Can you work these out from the model? Positions are in its coordinate system, mm. A direction names the side the tool comes from. Round coordinates to 2 decimals unless told otherwise and drop trailing zeros. Write each loop counter-clockwise with the first axis right and the second up, starting at its lowest first coordinate (ties: lowest second). Pieces come first, ordered by that corner, then holes.
Q1. For faces 1 (the flat face through (0, 37.5, 13)), 2 (the flat face through (14.5, 1, 5)), 3 (the flat face through (-14, -39.5, 7)), which set-ups out of +Z, -Z, +X, -X, +Y, -Y let a thin tool reach every point of the face, with its end or its side?
Q2. I'm going to push flat-ended pins straight in: pin 1 Ø1.6 at (x, y) = (-13.5, -1) entering from +Z; pin 2 Ø10 at (x, y) = (4.5, 19) entering from +Z; pin 3 Ø1.2 at (x, z) = (-8.47, 12.5) entering from -Y; pin 4 Ø1 at (x, z) = (-13, 6) entering from -Y. Where does each tip first touch, or does it pass through?
Q3. Please list where these lines run through material, in increasing order: line 1 along Y through (x, z) = (0, -0.55); line 2 along X through (y, z) = (7, 5.5); line 3 along Z through (x, y) = (1.75, 24.5).
Q4. If we section it at A-A (y = 34.5): Please give me the cut outline in (x, z).
Q5. We'd pull the mould along X, two halves only. Please class faces 4 (the cylindrical face through (0, -48, -1)), 5 (the flat face through (14, -39.5, 7)), 6 (the flat face through (-14.5, 1, 5)): +X half, -X half, draft (parallel to the pull), parting line (faces both ways), or undercut.
Q6. If we section it at B-B (x = 0): Please give me the cut outline in (y, z), plus the area to 3 significant figures.
Q7. If we section it at C-C (z = 10): Please give me the cut outline in (x, y), plus the area to 3 significant figures.
Q8. If we section it at D-D (x = 8.5): Please give me the cut outline in (y, z).
from build123d import *

# Parameters (mm, degrees)
ESQUISSE1_R             = 1
BOSS_EXTRU_2_DEPTH      = 2
ESQUISSE4_W             = 12.5
ESQUISSE4_H             = 79
BOSS_EXTRU_3_DEPTH      = 2
ESQUISSE6_W             = 12.5
ESQUISSE6_H             = 79
BOSS_EXTRU_4_DEPTH      = 2
BOSS_EXTRU_7_DEPTH      = 2
ESQUISSE14_R            = 1
ENL_V_MAT_EXTRU_4_DEPTH = 98.864702523
CHANFREIN3_SIZE         = 0.5
CONG_1_R                = 1


with BuildPart() as part:
    # Esquisse1 → Boss.-Extru.2 (new body)
    with BuildSketch(Plane.XY):
        with BuildLine():
            Line((14.5, -39.5), (14.5, 39.5))
            Line((14.5, 39.5), (-14.5, 39.5))
            Line((-14.5, 39.5), (-14.5, -39.5))
            ThreePointArc((-14.5, -39.5), (0, -54), (14.5, -39.5))
        make_face()
        with Locations((0, 34.5)):
            Circle(ESQUISSE1_R, mode=Mode.SUBTRACT)
        with Locations((0, -49)):
            Circle(ESQUISSE1_R, mode=Mode.SUBTRACT)
    extrude(amount=-BOSS_EXTRU_2_DEPTH)

    # Esquisse4 → Boss.-Extru.3 (add)
    with BuildSketch(Plane.ZY.offset(14.5)):
        with Locations((6.25, 0)):
            Rectangle(ESQUISSE4_W, ESQUISSE4_H)
    extrude(amount=-BOSS_EXTRU_3_DEPTH)

    # Esquisse6 → Boss.-Extru.4 (add)
    with BuildSketch(Plane(origin=(14.5, 0, 0), x_dir=(0, 0, -1), z_dir=(1, 0, 0))):
        with Locations((-6.25, 0)):
            Rectangle(ESQUISSE6_W, ESQUISSE6_H)
    extrude(amount=-BOSS_EXTRU_4_DEPTH)

    # Esquisse11 → Boss.-Extru.7 (add)
    with BuildSketch(Plane(origin=(0, 39.5, 0), x_dir=(1, 0, 0), z_dir=(0, 1, 0))):
        with BuildLine():
            Line((-12.5, 0), (12.5, 0))
            Line((12.5, 0), (12.5, -12.5))
            ThreePointArc((12.5, -12.5), (0, -25), (-12.5, -12.5))
            Line((-12.5, -12.5), (-12.5, 0))
        make_face()
    extrude(amount=-BOSS_EXTRU_7_DEPTH)

    # Esquisse14 → Enlèv. mat.-Extru.4 (cut, through all)
    with BuildSketch(Plane(origin=(0, 39.5, 0), x_dir=(1, 0, 0), z_dir=(0, 1, 0))):
        with Locations(Location((-8.474453363, -12.5, 0), (0, 0, 270))):
            Circle(ESQUISSE14_R)
        with Locations(Location((8.5, -12.5, 0), (0, 0, 270))):
            Circle(ESQUISSE14_R)
    extrude(amount=-ENL_V_MAT_EXTRU_4_DEPTH, mode=Mode.SUBTRACT)

    # Chanfrein3
    chanfrein3_edges = [part.edges().sort_by_distance(p)[0] for p in [
        (-12.5, -1, 12.5),
        (12.5, -1, 12.5),
    ]]
    chamfer(chanfrein3_edges, length=CHANFREIN3_SIZE)

    # Congé1
    # the kernel refuses this fillet: 1 mm, written as the material it adds along each edge
    with BuildSketch(Plane(origin=(-14.5, -39.5, 0), x_dir=(0, -1, 0), z_dir=(1, 0, 0))) as cong_1_piece_1_section:
        with BuildLine():
            CenterArc((CONG_1_R, -CONG_1_R), CONG_1_R, 90, 90)
            Line((0, -CONG_1_R), (-CONG_1_R * 0.02, -CONG_1_R))
            Line((-CONG_1_R * 0.02, -CONG_1_R), (-CONG_1_R * 0.02, CONG_1_R * 0.02))
            Line((-CONG_1_R * 0.02, CONG_1_R * 0.02), (CONG_1_R, CONG_1_R * 0.02))
            Line((CONG_1_R, CONG_1_R * 0.02), (CONG_1_R, 0))
        make_face()
    cong_1_piece_1 = extrude(amount=2, mode=Mode.PRIVATE)
    cong_1_piece_1 = cong_1_piece_1 & Plane(origin=(0, -39.5, 0.22667443), x_dir=(-1, 0, 0), z_dir=(0, 0, 1)) * Cylinder(14.5, 8, mode=Mode.PRIVATE)
    add(cong_1_piece_1)
    with BuildSketch(Plane(origin=(12.5, -39.5, 0), x_dir=(0, 0, 1), z_dir=(0, 1, 0)), Plane(origin=(-12.5, -39.5, 0), x_dir=(1, 0, 0), z_dir=(0, 1, 0))) as cong_1_piece_2:
        with BuildLine():
            CenterArc((CONG_1_R, -CONG_1_R), CONG_1_R, 90, 90)
            Line((0, -CONG_1_R), (-CONG_1_R * 0.02, -CONG_1_R))
            Line((-CONG_1_R * 0.02, -CONG_1_R), (-CONG_1_R * 0.02, CONG_1_R * 0.02))
            Line((-CONG_1_R * 0.02, CONG_1_R * 0.02), (CONG_1_R, CONG_1_R * 0.02))
            Line((CONG_1_R, CONG_1_R * 0.02), (CONG_1_R, 0))
        make_face()
    extrude(amount=77)
    with BuildSketch(Plane(origin=(14.5, -39.5, 0), x_dir=(0, 0, 1), z_dir=(-1, 0, 0))) as cong_1_piece_3_section:
        with BuildLine():
            CenterArc((CONG_1_R, -CONG_1_R), CONG_1_R, 90, 90)
            Line((0, -CONG_1_R), (-CONG_1_R * 0.02, -CONG_1_R))
            Line((-CONG_1_R * 0.02, -CONG_1_R), (-CONG_1_R * 0.02, CONG_1_R * 0.02))
            Line((-CONG_1_R * 0.02, CONG_1_R * 0.02), (CONG_1_R, CONG_1_R * 0.02))
            Line((CONG_1_R, CONG_1_R * 0.02), (CONG_1_R, 0))
        make_face()
    cong_1_piece_3 = extrude(amount=2, mode=Mode.PRIVATE)
    cong_1_piece_3 = cong_1_piece_3 & Plane(origin=(0, -39.5, 0.226674419), x_dir=(-1, 0, 0), z_dir=(0, 0, 1)) * Cylinder(14.5, 8, mode=Mode.PRIVATE)
    add(cong_1_piece_3)
    with BuildSketch(Plane(origin=(-12.5, 37.5, 0), x_dir=(0, 0, 1), z_dir=(1, 0, 0))) as cong_1_piece_4:
        with BuildLine():
            CenterArc((CONG_1_R, CONG_1_R), CONG_1_R, 180, 90)
            Line((0, CONG_1_R), (-CONG_1_R * 0.02, CONG_1_R))
            Line((-CONG_1_R * 0.02, CONG_1_R), (-CONG_1_R * 0.02, -CONG_1_R * 0.02))
            Line((-CONG_1_R * 0.02, -CONG_1_R * 0.02), (CONG_1_R, -CONG_1_R * 0.02))
            Line((CONG_1_R, -CONG_1_R * 0.02), (CONG_1_R, 0))
        make_face()
    extrude(amount=25)
    with BuildSketch(Plane(origin=(-14.5, -39.5, 0), x_dir=(0, -1, 0), z_dir=(1, 0, 0))) as cong_1_piece_5a_section:
        with BuildLine():
            CenterArc((CONG_1_R, -CONG_1_R), CONG_1_R, 90, 90)
            Line((0, -CONG_1_R), (-CONG_1_R * 0.02, -CONG_1_R))
            Line((-CONG_1_R * 0.02, -CONG_1_R), (-CONG_1_R * 0.02, CONG_1_R * 0.02))
            Line((-CONG_1_R * 0.02, CONG_1_R * 0.02), (CONG_1_R, CONG_1_R * 0.02))
            Line((CONG_1_R, CONG_1_R * 0.02), (CONG_1_R, 0))
        make_face()
    cong_1_piece_5a = extrude(amount=4.5, mode=Mode.PRIVATE)
    cong_1_piece_5a = split(cong_1_piece_5a, bisect_by=Plane(origin=(-12.5, -39.726395114, 0.226395114), z_dir=(1, 0, 0)), keep=Keep.TOP, mode=Mode.PRIVATE)
    with BuildSketch(Plane(origin=(-12.5, -42, 0), x_dir=(1, 0, 0), z_dir=(0, 1, 0))) as cong_1_piece_5b_section:
        with BuildLine():
            CenterArc((CONG_1_R, -CONG_1_R), CONG_1_R, 90, 90)
            Line((0, -CONG_1_R), (-CONG_1_R * 0.02, -CONG_1_R))
            Line((-CONG_1_R * 0.02, -CONG_1_R), (-CONG_1_R * 0.02, CONG_1_R * 0.02))
            Line((-CONG_1_R * 0.02, CONG_1_R * 0.02), (CONG_1_R, CONG_1_R * 0.02))
            Line((CONG_1_R, CONG_1_R * 0.02), (CONG_1_R, 0))
        make_face()
    cong_1_piece_5b = extrude(amount=79.5, mode=Mode.PRIVATE)
    cong_1_piece_5b = split(cong_1_piece_5b, bisect_by=Plane(origin=(-12.273604886, -39.5, 0.226395114), z_dir=(0, -1, 0)), keep=Keep.TOP, mode=Mode.PRIVATE)
    cong_1_piece_5 = cong_1_piece_5a & cong_1_piece_5b
    add(cong_1_piece_5)
    with BuildSketch(Plane(origin=(14.5, -39.5, 0), x_dir=(0, 0, 1), z_dir=(-1, 0, 0))) as cong_1_piece_6a_section:
        with BuildLine():
            CenterArc((CONG_1_R, -CONG_1_R), CONG_1_R, 90, 90)
            Line((0, -CONG_1_R), (-CONG_1_R * 0.02, -CONG_1_R))
            Line((-CONG_1_R * 0.02, -CONG_1_R), (-CONG_1_R * 0.02, CONG_1_R * 0.02))
            Line((-CONG_1_R * 0.02, CONG_1_R * 0.02), (CONG_1_R, CONG_1_R * 0.02))
            Line((CONG_1_R, CONG_1_R * 0.02), (CONG_1_R, 0))
        make_face()
    cong_1_piece_6a = extrude(amount=4.5, mode=Mode.PRIVATE)
    cong_1_piece_6a = split(cong_1_piece_6a, bisect_by=Plane(origin=(12.5, -39.726395114, 0.226395114), z_dir=(-1, 0, 0)), keep=Keep.TOP, mode=Mode.PRIVATE)
    with BuildSketch(Plane(origin=(12.5, -42, 0), x_dir=(0, 0, 1), z_dir=(0, 1, 0))) as cong_1_piece_6b_section:
        with BuildLine():
            CenterArc((CONG_1_R, -CONG_1_R), CONG_1_R, 90, 90)
            Line((0, -CONG_1_R), (-CONG_1_R * 0.02, -CONG_1_R))
            Line((-CONG_1_R * 0.02, -CONG_1_R), (-CONG_1_R * 0.02, CONG_1_R * 0.02))
            Line((-CONG_1_R * 0.02, CONG_1_R * 0.02), (CONG_1_R, CONG_1_R * 0.02))
            Line((CONG_1_R, CONG_1_R * 0.02), (CONG_1_R, 0))
        make_face()
    cong_1_piece_6b = extrude(amount=79.5, mode=Mode.PRIVATE)
    cong_1_piece_6b = split(cong_1_piece_6b, bisect_by=Plane(origin=(12.273604886, -39.5, 0.226395114), z_dir=(0, -1, 0)), keep=Keep.TOP, mode=Mode.PRIVATE)
    cong_1_piece_6 = cong_1_piece_6a & cong_1_piece_6b
    add(cong_1_piece_6)
    with BuildSketch(Plane(origin=(-12.5, 37.5, 0), x_dir=(0, 0, 1), z_dir=(1, 0, 0))) as cong_1_piece_7a_section:
        with BuildLine():
            CenterArc((CONG_1_R, CONG_1_R), CONG_1_R, 180, 90)
            Line((0, CONG_1_R), (-CONG_1_R * 0.02, CONG_1_R))
            Line((-CONG_1_R * 0.02, CONG_1_R), (-CONG_1_R * 0.02, -CONG_1_R * 0.02))
            Line((-CONG_1_R * 0.02, -CONG_1_R * 0.02), (CONG_1_R, -CONG_1_R * 0.02))
            Line((CONG_1_R, -CONG_1_R * 0.02), (CONG_1_R, 0))
        make_face()
    cong_1_piece_7a = extrude(amount=27.5, mode=Mode.PRIVATE)
    cong_1_piece_7a = split(cong_1_piece_7a, bisect_by=Plane(origin=(12.5, 37.273604886, 0.226395114), z_dir=(1, 0, 0)), keep=Keep.TOP, mode=Mode.PRIVATE)
    with BuildSketch(Plane(origin=(12.5, -39.5, 0), x_dir=(0, 0, 1), z_dir=(0, 1, 0))) as cong_1_piece_7b_section:
        with BuildLine():
            CenterArc((CONG_1_R, -CONG_1_R), CONG_1_R, 90, 90)
            Line((0, -CONG_1_R), (-CONG_1_R * 0.02, -CONG_1_R))
            Line((-CONG_1_R * 0.02, -CONG_1_R), (-CONG_1_R * 0.02, CONG_1_R * 0.02))
            Line((-CONG_1_R * 0.02, CONG_1_R * 0.02), (CONG_1_R, CONG_1_R * 0.02))
            Line((CONG_1_R, CONG_1_R * 0.02), (CONG_1_R, 0))
        make_face()
    cong_1_piece_7b = extrude(amount=79.5, mode=Mode.PRIVATE)
    cong_1_piece_7b = split(cong_1_piece_7b, bisect_by=Plane(origin=(12.273604886, 37.5, 0.226395114), z_dir=(0, 1, 0)), keep=Keep.TOP, mode=Mode.PRIVATE)
    cong_1_piece_7 = cong_1_piece_7a & cong_1_piece_7b
    add(cong_1_piece_7)
    with BuildSketch(Plane(origin=(-15, 37.5, 0), x_dir=(0, 0, 1), z_dir=(1, 0, 0))) as cong_1_piece_8a_section:
        with BuildLine():
            CenterArc((CONG_1_R, CONG_1_R), CONG_1_R, 180, 90)
            Line((0, CONG_1_R), (-CONG_1_R * 0.02, CONG_1_R))
            Line((-CONG_1_R * 0.02, CONG_1_R), (-CONG_1_R * 0.02, -CONG_1_R * 0.02))
            Line((-CONG_1_R * 0.02, -CONG_1_R * 0.02), (CONG_1_R, -CONG_1_R * 0.02))
            Line((CONG_1_R, -CONG_1_R * 0.02), (CONG_1_R, 0))
        make_face()
    cong_1_piece_8a = extrude(amount=27.5, mode=Mode.PRIVATE)
    cong_1_piece_8a = split(cong_1_piece_8a, bisect_by=Plane(origin=(-12.5, 37.273604886, 0.226395114), z_dir=(-1, 0, 0)), keep=Keep.TOP, mode=Mode.PRIVATE)
    with BuildSketch(Plane(origin=(-12.5, -39.5, 0), x_dir=(1, 0, 0), z_dir=(0, 1, 0))) as cong_1_piece_8b_section:
        with BuildLine():
            CenterArc((CONG_1_R, -CONG_1_R), CONG_1_R, 90, 90)
            Line((0, -CONG_1_R), (-CONG_1_R * 0.02, -CONG_1_R))
            Line((-CONG_1_R * 0.02, -CONG_1_R), (-CONG_1_R * 0.02, CONG_1_R * 0.02))
            Line((-CONG_1_R * 0.02, CONG_1_R * 0.02), (CONG_1_R, CONG_1_R * 0.02))
            Line((CONG_1_R, CONG_1_R * 0.02), (CONG_1_R, 0))
        make_face()
    cong_1_piece_8b = extrude(amount=79.5, mode=Mode.PRIVATE)
    cong_1_piece_8b = split(cong_1_piece_8b, bisect_by=Plane(origin=(-12.273604886, 37.5, 0.226395114), z_dir=(0, 1, 0)), keep=Keep.TOP, mode=Mode.PRIVATE)
    cong_1_piece_8 = cong_1_piece_8a & cong_1_piece_8b
    add(cong_1_piece_8)


solid = part.part
A:
1. face 1: +Z, -Y
1. face 2: +Z, -Z, +X, +Y, -Y
1. face 3: +Z, +X, -X, -Y
2. pin 1: stops at z = 12.5
2. pin 2: stops at z = 0
2. pin 3: passes through
2. pin 4: stops at y = -39.5
3. line 1: y = -54 to -50, -48 to 33.5, 35.5 to 39.5
3. line 2: x = -14.5 to -12.5, 12.5 to 14.5
3. line 3: z = -2 to 0
4. outline: (-14.5, -2) - (-1, -2) - (-1, 0) - (-11.5, 0) arc R1 cw to (-12.5, 1) - (-12.5, 12) - (-13, 12.5) - (-14.5, 12.5) - close; (1, -2) - (14.5, -2) - (14.5, 12.5) - (13, 12.5) - (12.5, 12) - (12.5, 1) arc R1 cw to (11.5, 0) - (1, 0) - close
5. face 4: undercut
5. face 5: draft
5. face 6: -X half
6. outline: (-54, -2) - (-50, -2) - (-50, 0) - (-54, 0) - close; (-48, -2) - (33.5, -2) - (33.5, 0) - (-48, 0) - close; (35.5, -2) - (39.5, -2) - (39.5, 25) - (37.5, 25) - (37.5, 1) arc R1 cw to (36.5, 0) - (35.5, 0) - close
6. area: 229 mm2
7. outline: (-14.5, -39.5) - (-12.5, -39.5) - (-12.5, 37.5) - (12.5, 37.5) - (12.5, -39.5) - (14.5, -39.5) - (14.5, 39.5) - (-14.5, 39.5) - close
7. area: 366 mm2
8. outline: (-51.25, -2) - (39.5, -2) - (39.5, 11.5) - (37.5, 11.5) - (37.5, 1) arc R1 cw to (36.5, 0) - (-51.25, 0) - close; (37.5, 13.5) - (39.5, 13.5) - (39.5, 21.67) - (37.5, 21.67) - close
